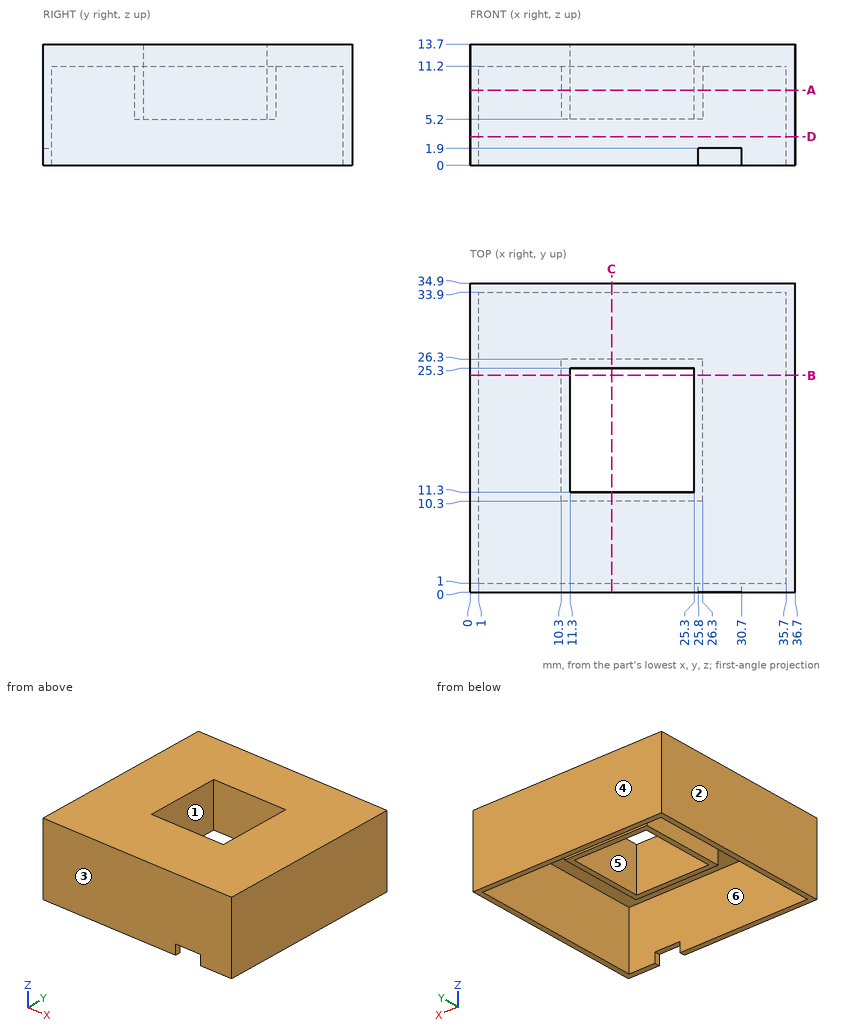
Study the drawing (mm; zero at the part's minimum x, y, z) and answer. A direction names the side the tool comes from. Round coordinates to 2 decimals unless told otherwise and drop trailing zeros. Loops run counter-clockwise (first coordinate to the right, second up) from the corner with the lowest first, then second, coordinate; pieces in that order, holes last. Notation, with made-up numbers: (34, -27) -> (63, -27) arc R18 cw to (63, 1) -> close; hole circle Ø3 at (82.25, 36). An arc over 180 degrees is marked (long way). Use one line per item in the form item = value.
1. For a pull along Y with two mould halves and no side action, classify the marked faces 1, 2 and 3 as released by +Y, released by -Y, zero draft, split by the parting line, or undercut.
Answer key:
face_1 = undercut
face_2 = zero draft
face_3 = released by -Y
2. The part is cut by section C-C on x = 16. Determine the outline of the cut face in (y, z), and give its area (4 significant figures).
Answer key:
outline = (0, 0) -> (1, 0) -> (1, 11.2) -> (10.3, 11.2) -> (10.3, 5.2) -> (11.3, 5.2) -> (11.3, 13.7) -> (0, 13.7) -> close; (25.3, 5.2) -> (26.3, 5.2) -> (26.3, 11.2) -> (33.9, 11.2) -> (33.9, 0) -> (34.9, 0) -> (34.9, 13.7) -> (25.3, 13.7) -> close
area = 86.65 mm²
3. Find the intervals of material crossed by probe 1 along Y at (x, z) = (26, 9); probe 2 along Y at (x, z) = (21, 9.25); probe 3 along X at (y, z) = (21.5, 6.5), in increasing order. Write a range as [from, to].
Answer key:
probe_1 = [0, 1], [10.3, 26.3], [33.9, 34.9]
probe_2 = [0, 1], [10.3, 11.3], [25.3, 26.3], [33.9, 34.9]
probe_3 = [0, 1], [10.3, 11.3], [25.3, 26.3], [35.7, 36.7]
4. The part is cut by section D-D on z = 3.25. Determine the outline of the cut face in (x, y), and give its area (3 significant figures).
Answer key:
outline = (0, 0) -> (36.7, 0) -> (36.7, 34.9) -> (0, 34.9) -> close; hole (1, 1) -> (35.7, 1) -> (35.7, 33.9) -> (1, 33.9) -> close
area = 139 mm²
5. A tool of negligible diameter and unlimited length cuts with its end or side. For the marked faces 4, 5 and 6, from which of +Z, -Z, +X, -X, +Y, -Y can it reach the whole face along a straight path? Write none if from no direction.
Answer key:
face_4 = +Z, -Z, +X, -X, +Y
face_5 = +Z, -Z
face_6 = -Z
6. The part is cut by section A-A on z = 8.5. Determine the outline of the cut face in (x, y).
Answer key:
outline = (0, 0) -> (36.7, 0) -> (36.7, 34.9) -> (0, 34.9) -> close; (10.3, 10.3) -> (26.3, 10.3) -> (26.3, 26.3) -> (10.3, 26.3) -> close; hole (1, 1) -> (35.7, 1) -> (35.7, 33.9) -> (1, 33.9) -> close; hole (11.3, 11.3) -> (25.3, 11.3) -> (25.3, 25.3) -> (11.3, 25.3) -> close
7. The part is cut by section B-B on y = 24.5. Determine the outline of the cut face in (x, z).
Answer key:
outline = (0, 0) -> (1, 0) -> (1, 11.2) -> (10.3, 11.2) -> (10.3, 5.2) -> (11.3, 5.2) -> (11.3, 13.7) -> (0, 13.7) -> close; (25.3, 5.2) -> (26.3, 5.2) -> (26.3, 11.2) -> (35.7, 11.2) -> (35.7, 0) -> (36.7, 0) -> (36.7, 13.7) -> (25.3, 13.7) -> close
8. Flat-ended cylindrical pins translate along their axes: pin 1 Ø1 at (x, y) = (19.5, 12.5) entering from -Z; pin 2 Ø6 at (x, y) = (31.5, 14.5) entering from -Z; pin 3 Ø3 at (x, y) = (15, 10.5) entering from -Z; pin 4 Ø1.1 at (x, y) = (28.5, 0.5) entering from -Z. Find the tip coordinate at first contact, or state that the pin passes through.
Answer key:
pin_1 = through
pin_2 = 11.2
pin_3 = 5.2
pin_4 = 1.9
